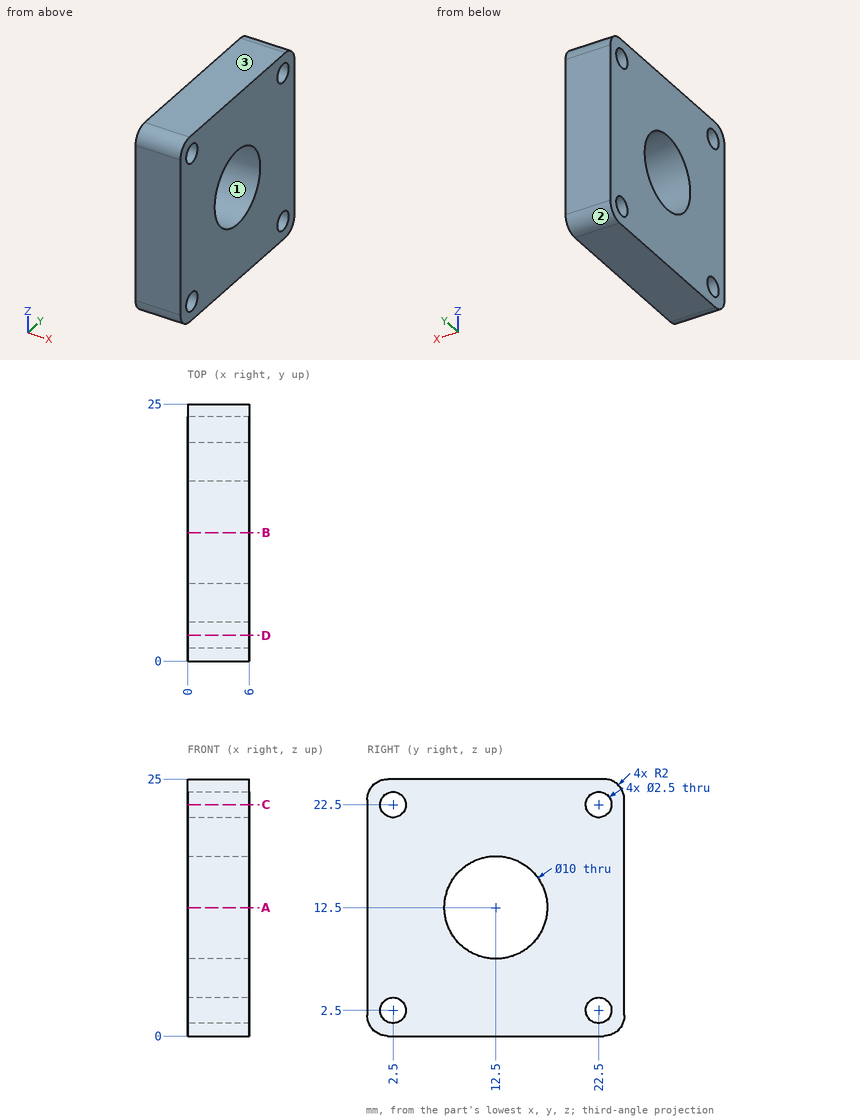
Could you check a few things on this drawing? It's one solid part, dimensions in mm from its lowest x, y, z. Round coordinates to 2 decimals unless told otherwise and drop trailing zeros. Order: outer loops, then holes, each group sorted by start corner. A loop starts at its lowest first (then second) coordinate and runs counter-clockwise, first axis right, second up. Notation, with made-up numbers: M 79.5,43.5 L 125.5,43.5 A32 ccw 125.5,73.5 Z; hole C -7.75,36.5 d10. An arc over 180 degrees is marked long. One line per item, written item: value.
(1) Imagine slicing it at A-A (z = 12.5). Write out the boundary of the cut face in (x, y).
Ans:
outline: M 0,0 L 6,0 L 6,7.5 L 0,7.5 Z; M 0,17.5 L 6,17.5 L 6,25 L 0,25 Z
(2) I need wall thicknesses on line 1 along Y through (x, z) = (3.3, 22.5); line 2 along Y through (x, z) = (2.1, 23); line 3 along Y through (x, z) = (4.5, 12.5). Which ranges of each line are inside material? Lowest first, please. Write a range as from..to.
Ans:
line 1: y = 0..1.25, 3.75..21.25, 23.75..25
line 2: y = 0..1.35, 3.65..21.35, 23.65..25
line 3: y = 0..7.5, 17.5..25
(3) If we mould it in two halves opening along Z, with no side actions, what happens to the marked faces 1, 2 and 3? For each: released by +Z, released by -Z, zero draft, split by the parting line, or undercut.
Ans:
face 1: undercut
face 2: released by -Z
face 3: released by +Z
(4) Imagine slicing it at C-C (z = 22.5). Write out the boundary of the cut face in (x, y).
Ans:
outline: M 0,0 L 6,0 L 6,1.25 L 0,1.25 Z; M 0,3.75 L 6,3.75 L 6,21.25 L 0,21.25 Z; M 0,23.75 L 6,23.75 L 6,25 L 0,25 Z
